Could you check a few things on this drawing? It's one solid part, dimensions in mm from its lowest x, y, z. Round coordinates to 2 decimals unless told otherwise and drop trailing zeros. Write each loop counter-clockwise with the first axis right and the second up, starting at its lowest first coordinate (ties: lowest second). Pieces come first, ordered by that corner, then holes. Notation, with made-up numbers: M 11,-27 L 58,-27 A11 cw 58,-6 Z; hole C 45,52 d2. An arc over 180 degrees is marked long. One line per item, written item: value. Start each with the question number.
(1) I want a section at D-D on y = 16.5. Please give me the cut outline in (x, z), and give its area (3 significant figures).
(2) I want a section at C-C on z = 0.7. Please give me the cut outline in (x, y) (1 decimal), and give its area (3 significant figures).
(3) I'm going to push flat-ended pins straight in: pin 1 Ø1.5 at (x, z) = (72.5, 1.5) entering from -Y; pin 2 Ø1.6 at (x, z) = (67.5, 2.5) entering from -Y; pin 3 Ø0.9 at (x, z) = (64, 2) entering from +Y; pin 4 Ø8 at (x, y) = (34, 13) entering from -Z. Where does each tip first touch, or does it pass through?
(4) If I drill on L1, parallel to Y at x = 57, z = 1.05; L2, parallel to Z at x = 49, y = 14; L3, parallel to Y at x = 29.5, z = 1.4, over which ranges is the centre line in solid material (lowest first)?
(5) I want a section at B-B on y = 8. Please give me the cut outline in (x, z) (1 decimal), and give its area (3 significant figures).
(6) I want a section at A-A on x = 64. Please give me the cut outline in (y, z), and give its area (3 significant figures).
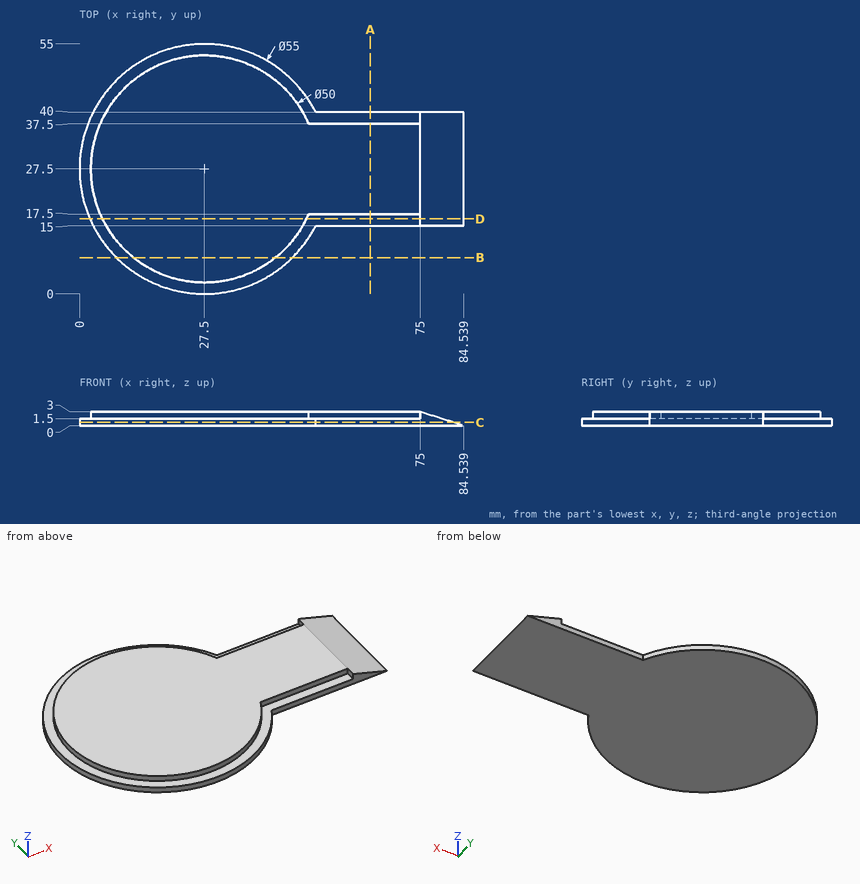
Found:
1. outline: M 2.3,0 L 84.54,0 L 75,3 L 75,1.5 L 49.95,1.5 L 49.95,3 L 5.05,3 L 5.05,1.5 L 2.3,1.5 Z
1. area: 191 mm²
2. outline: M 52,15 L 82.3,15 L 82.3,40 L 52,40 A27.5 ccw long Z
2. area: 3,080 mm²
3. pin 1: stops at y = 15
3. pin 2: stops at y = 17.5
3. pin 3: stops at y = 37.5
3. pin 4: stops at z = 0
4. L1: y = 15 to 40
4. L2: z = 0 to 1.5
4. L3: y = 0.07 to 54.93
5. outline: M 8.1,0 L 46.9,0 L 46.9,1.5 L 43.1,1.5 L 43.1,3 L 11.9,3 L 11.9,1.5 L 8.1,1.5 Z
5. area: 105 mm²
6. outline: M 15,0 L 40,0 L 40,1.5 L 37.5,1.5 L 37.5,3 L 17.5,3 L 17.5,1.5 L 15,1.5 Z
6. area: 67.5 mm²
